Could you check a few things on this model? Use its own coordinates, in mm. Round coordinates to 2 decimals unless told otherwise and drop trailing zeros. Loops run counter-clockwise (first coordinate to the right, second up) from the corner with the lowest first, then second, coordinate; pieces in that order, holes last.
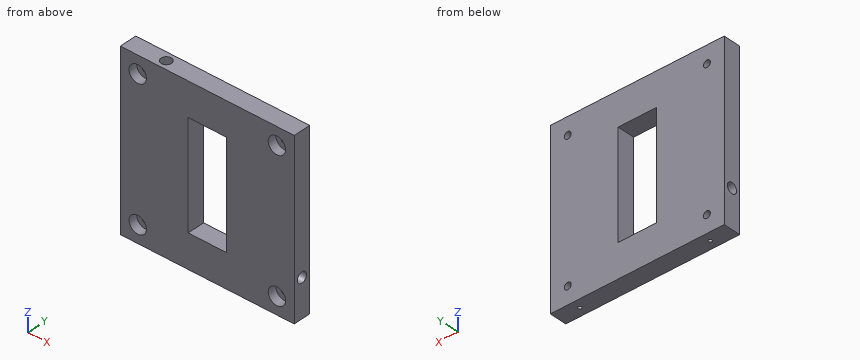
Autodesk Inventor part; units mm, degrees
ref_plane "YZ Plane" through (0, 0, 0) normal (1, 0, 0) x (0, 1, 0)
ref_plane "XZ Plane" through (0, 0, 0) normal (0, 1, 0) x (-1, 0, 0)
ref_plane "XY Plane" through (0, 0, 0) normal (0, 0, 1) x (1, 0, 0)
sketch "Szkic1" plane through (0, 0, 0) normal (0, 1, 0) x (-1, 0, 0)
  line L0 (25, 25) -> (-25, 25)
  line L1 (-25, 25) -> (-25, -25)
  line L2 (-25, -25) -> (25, -25)
  line L3 (25, -25) -> (25, 25)
  line L4 (0, 25) -> (0, -25)
  line L5 (25, 0) -> (-25, 0)
  circle A0 centre (20, -20) radius 2.5
  circle A1 centre (20, 20) radius 2.5
  circle A2 centre (-20, -20) radius 2.5
  circle A3 centre (-20, 20) radius 2.5
  line L6 (-5.5, 15.3) -> (5.5, 15.3)
  line L7 (5.5, 15.3) -> (5.5, -15.3)
  line L8 (5.5, -15.3) -> (-5.5, -15.3)
  line L9 (-5.5, -15.3) -> (-5.5, 15.3)
  point P0 (0, 0)
  point P1 (0, 0)
  dimension "d0" = 50
  dimension "d1" = 50
  dimension "d2" = 25
  dimension "d3" = 25
  dimension "d4" = 5
  dimension "d5" = 20
  dimension "d6" = 20
  dimension "d69" = 11
  dimension "d70" = 30.6
sketch "Szkic2" plane through (0, 0, 0) normal (0, 1, 0) x (-1, 0, 0)
  point P0 (0, 0)
extrude "Wyciągnięcie proste1" add sketch "Szkic1" along normal blind 5 contours L3 L5 L7 L6 L4 L0 | L4 L6 L9 L5 L1 L0 | L3 L2 L4 L8 L7 L5 | L5 L9 L8 L4 L2 L1 | A0 | A1 | A2 | A3
sketch "Szkic3" plane through (0, 0, 0) normal (0, -1, 0) x (1, 0, 0)
  circle A0 centre (-20, -20) radius 2.5
  line L0 (0, 29.2243) -> (0, -29.2243)
  line L1 (55.447, 0) -> (-42.023, 0)
  circle A1 centre (20, -20) radius 2.5
  circle A2 centre (-20, 20) radius 2.5
  circle A3 centre (20, 20) radius 2.5
  point P0 (0, 0)
  point P1 (0, 0)
  dimension "d9" = 5
  dimension "d10" = 20
  dimension "d11" = 20
hole "Otwór1" at (20, 0, -20) at (-20, 0, -20) at (-20, 0, 20) at (20, 0, 20) direction (0, 1, 0) diameter 5 depth 2.5
sketch "Szkic4" plane through (0, 5, 0) normal (0, 1, 0) x (1, 0, 0)
  line L0 (53.1876, 0) -> (-53.1876, 0)
  line L1 (0, 32.3787) -> (0, -30.0481)
  circle A0 centre (20, -20) radius 2.5
  circle A1 centre (20, -20) radius 2.5
  circle A2 centre (-20, -20) radius 2.5
  circle A3 centre (20, 20) radius 2.5
  circle A4 centre (20, 20) radius 2.5
  circle A5 centre (-20, 20) radius 2.5
  circle A6 centre (-20, 20) radius 2.5
  point P0 (0, 0)
  point P1 (0, 0)
hole "Otwór2" at (-20, 5, -20) at (20, 5, -20) at (20, 5, 20) at (-20, 5, 20) direction (0, -1, 0) diameter 2 depth 2.5
sketch "Szkic5" plane through (25, 0, 25) normal (1, 0, 0) x (0, 0, -1)
  circle A0 centre (39, 2.5) radius 1.5
  line L0 (0, 0) -> (50, 0)
  line L1 (50, 0) -> (50, 5)
  point P0 (25, 0)
  dimension "d26" = 3
  dimension "d27" = 2.5
  dimension "d28" = 11
sketch "Szkic6" plane through (-25, 0, -25) normal (-1, 0, 0) x (0, 0, 1)
  circle A0 centre (11, 2.5) radius 1.5
  line L0 (0, 0) -> (0, 5)
  line L1 (0, 0) -> (50, 0)
  point P0 (25, 0)
  dimension "d29" = 3
  dimension "d30" = 11
  dimension "d31" = 2.5
sketch "Szkic7" plane through (-25, 0, 25) normal (0, 0, 1) x (1, 0, 0)
  circle A0 centre (11, 2.5) radius 1.5
  line L0 (0, 0) -> (0, 5)
  line L1 (0, 0) -> (50, 0)
  point P0 (25, 0)
  dimension "d32" = 3
  dimension "d33" = 11
  dimension "d34" = 2.5
hole "Otwór3" at (-14, 2.5, 25) direction (0, 0, -1) diameter 3 depth 3
hole "Otwór4" at (-25, 2.5, -14) direction (1, 0, 0) diameter 3 depth 3
hole "Otwór5" at (25, 2.5, -14) direction (-1, 0, 0) diameter 3 depth 3
sketch "Szkic8" plane through (25, 0, -25) normal (0, 0, -1) x (-1, 0, 0)
  circle A0 centre (6.25, 2.5) radius 0.5
  line L0 (0, 0) -> (0, 5)
  line L1 (0, 0) -> (50, 0)
  circle A1 centre (43.75, 2.5) radius 0.5
  line L2 (50, 0) -> (50, 5)
  point P0 (25, 0)
  dimension "d56" = 6.25
  dimension "d57" = 1
  dimension "d58" = 2.5
  dimension "d59" = 1
  dimension "d60" = 6.25
  dimension "d61" = 2.5
hole "Otwór6" at (18.75, 2.5, -25) at (-18.75, 2.5, -25) direction (0, 0, 1) diameter 1 depth 2.5
sketch "Szkic9" plane through (25, 0, 25) normal (1, 0, 0) x (0, 0, -1)
  point P0 (25, 0)
properties part number "platforma wriertnicza"
Item 1: If we section it at C-C, the plane z = 20: Please give me the cut outline in (x, y).
Results list:
outline: (-25, 0) - (-22.5, 0) - (-22.5, 2.5) - (-21, 2.5) - (-21, 5) - (-25, 5) - close; (-19, 2.5) - (-17.5, 2.5) - (-17.5, 0) - (17.5, 0) - (17.5, 2.5) - (19, 2.5) - (19, 5) - (-19, 5) - close; (21, 2.5) - (22.5, 2.5) - (22.5, 0) - (25, 0) - (25, 5) - (21, 5) - close
Item 2: Will these pins go through, and if not, where does the flat tip stop? pin 1 (4 mm diameter, centred on x = 20, z = -20, fed in from -Y); pin 2 (1.8 mm diameter, centred on y = 2.5, z = -14, fed in from +X); pin 3 (8 mm diameter, centred on x = 20, z = 20, fed in from -Y).
Results list:
pin 1: stops at y = 2.5
pin 2: stops at x = 22
pin 3: stops at y = 0
Item 3: If I drill on line 1 along X through (y, z) = (4.4, -20); line 2 along Z through (x, y) = (-4, 1.6); line 3 along X through (y, z) = (3.6, -10.5), over which ranges is the centre line in solid material (lowest first)?
Results list:
line 1: x = -25 to -21, -19 to 19, 21 to 25
line 2: z = -25 to -15.3, 15.3 to 25
line 3: x = -25 to -5.5, 5.5 to 25
Item 4: If we section it at B-B, the plane x = 20: Please give me the cut outline in (y, z), then the cut area to 3 significant figures.
Results list:
outline: (0, -25) - (5, -25) - (5, -21) - (2.5, -21) - (2.5, -22.5) - (0, -22.5) - close; (0, -17.5) - (2.5, -17.5) - (2.5, -19) - (5, -19) - (5, 19) - (2.5, 19) - (2.5, 17.5) - (0, 17.5) - close; (0, 22.5) - (2.5, 22.5) - (2.5, 21) - (5, 21) - (5, 25) - (0, 25) - close
area: 215 mm2
Item 5: If we section it at D-D, the plane z = 9: Please give me the cut outline in (x, y), then the cut area to 3 significant figures.
Results list:
outline: (-25, 0) - (-5.5, 0) - (-5.5, 5) - (-25, 5) - close; (5.5, 0) - (25, 0) - (25, 5) - (5.5, 5) - close
area: 195 mm2
Item 6: If we section it at A-A, the plane z = -14: Please give me the cut outline in (x, y), then the cut area to 3 significant figures.
Results list:
outline: (-25, 0) - (-5.5, 0) - (-5.5, 5) - (-25, 5) - (-25, 4) - (-22, 4) - (-22, 1) - (-25, 1) - close; (5.5, 0) - (25, 0) - (25, 1) - (22, 1) - (22, 4) - (25, 4) - (25, 5) - (5.5, 5) - close
area: 177 mm2
